```python
from build123d import *

# Parameters (mm, degrees)
SKETCH6_W           = 30
SKETCH6_H           = 25
BOSS_EXTRUDE6_DEPTH = 6
SKETCH7_W           = 15
SKETCH7_H           = 25
BOSS_EXTRUDE7_DEPTH = 3
SKETCH8_W           = 10
SKETCH8_H           = 10
BOSS_EXTRUDE8_DEPTH = 6
SKETCH9_W           = 25
SKETCH9_H           = 6
BOSS_EXTRUDE9_DEPTH = 15


with BuildPart() as part:
    # Sketch6 → Boss-Extrude6 (new body)
    with BuildSketch(Plane(origin=(0, 0, 0), x_dir=(1, 0, 0), z_dir=(0, 1, 0))):
        with Locations((-0.909090909, 0)):
            Rectangle(SKETCH6_W, SKETCH6_H)
    extrude(amount=BOSS_EXTRUDE6_DEPTH)

    # Sketch7 → Boss-Extrude7 (add)
    with BuildSketch(Plane(origin=(0, 6, 0), x_dir=(1, 0, 0), z_dir=(0, 1, 0))):
        with Locations((6.590909091, 0)):
            Rectangle(SKETCH7_W, SKETCH7_H)
    extrude(amount=BOSS_EXTRUDE7_DEPTH)

    # Sketch8 → Boss-Extrude8 (add)
    with BuildSketch(Plane(origin=(0, 6, 0), x_dir=(1, 0, 0), z_dir=(0, 1, 0))):
        with Locations((-10.909090909, 0)):
            Rectangle(SKETCH8_W, SKETCH8_H)
    extrude(amount=BOSS_EXTRUDE8_DEPTH)

    # Sketch9 → Boss-Extrude9 (add)
    with BuildSketch(Plane.ZY.offset(15.909090909)):
        with Locations((0, 3)):
            Rectangle(SKETCH9_W, SKETCH9_H)
    extrude(amount=BOSS_EXTRUDE9_DEPTH)


solid = part.part
```
Check sheet for the modelled part. Datum: model origin and axes. Units: mm. A direction names the side the tool comes from. Round coordinates to 2 decimals unless told otherwise and drop trailing zeros. Loops run counter-clockwise (first coordinate to the right, second up) from the corner with the lowest first, then second, coordinate; pieces in that order, holes last. Notation, with made-up numbers: (20, 70.25) -> (73, 70.25) arc R22 ccw to (73, 87.25) -> close; hole circle Ø6 at (46, 15.25). An arc over 180 degrees is marked (long way). Write item = value, one per line. Start each with the question number.
1) Sectioned sample at A-A, the plane y = 7.25. Record the cut outline in (x, z).
2) Release check for a two-part mould opening along X. For faces 6 (the flat face through (-0.909, 7, 0)), 7 (the flat face through (-30.909, 3, 0)), 8 (the flat face through (6, 9, 0)) record: released by +X, released by -X, zero draft, split by the parting line, or undercut.
3) Set-up check for faces 1 (the flat face through (-11, 9, -5)), 2 (the flat face through (-15.909, 9, 0)), 3 (the flat face through (-8, 3, -12.5)), 4 (the flat face through (-5.909, 9, 0)), 5 (the flat face through (-11, 9, 5)): record each of +Z, -Z, +X, -X, +Y, -Y from which the full face is reachable in a straight line by a thin tool's end or side.
4) Sectioned sample at B-B, the plane z = 3.25. Record the cut outline in (x, y), plus the area to 3 significant figures.
5) Sectioned sample at D-D, the plane y = 10. Record the cut outline in (x, z).
6) Sectioned sample at C-C, the plane x = -26.5. Record the cut outline in (y, z), plus the area to 3 significant figures.
7) Thickness scan on probe 1 along X at (y, z) = (8, -3); probe 2 along Y at (x, z) = (-29, -9); probe 3 along Z at (x, y) = (-6, 9.25). Record the ranges inside material, lowest first.
8) Gauge pin test, flat ends, axial feed: pin 1 Ø1.8 at (x, y) = (-10, 9.5) entering from -Z; pin 2 Ø4 at (x, z) = (3.5, -4) entering from +Y; pin 3 Ø3 at (x, y) = (-13, 8) entering from +Z. Record the tip position at first contact, or that the pin passes through.
Results are:
q1.outline = (-15.91, -5) -> (-5.91, -5) -> (-5.91, 5) -> (-15.91, 5) -> close; (-0.91, -12.5) -> (14.09, -12.5) -> (14.09, 12.5) -> (-0.91, 12.5) -> close
q2.face_6 = undercut
q2.face_7 = released by -X
q2.face_8 = zero draft
q3.face_1 = -Z, -X, +Y
q3.face_2 = +Z, -Z, -X, +Y
q3.face_3 = -Z, +X, -X, +Y, -Y
q3.face_4 = +Z, -Z, +Y
q3.face_5 = +Z, -X, +Y
q4.outline = (-30.91, 0) -> (14.09, 0) -> (14.09, 9) -> (-0.91, 9) -> (-0.91, 6) -> (-5.91, 6) -> (-5.91, 12) -> (-15.91, 12) -> (-15.91, 6) -> (-30.91, 6) -> close
q4.area = 375 mm^2
q5.outline = (-15.91, -5) -> (-5.91, -5) -> (-5.91, 5) -> (-15.91, 5) -> close
q6.outline = (0, -12.5) -> (6, -12.5) -> (6, 12.5) -> (0, 12.5) -> close
q6.area = 150 mm^2
q7.probe_1 = -15.91 to -5.91, -0.91 to 14.09
q7.probe_2 = 0 to 6
q7.probe_3 = -5 to 5
q8.pin_1 = -5
q8.pin_2 = 9
q8.pin_3 = 5
